Could you check a few things on this model? Use its own coordinates, in mm. Face numbers are marked on the shaded views. A direction names the side the tool comes from. Give positions to 0.01 mm unless a question says otherwise; leave off trailing zeros. Loops run counter-clockwise (first coordinate to the right, second up) from the corner with the lowest first, then second, coordinate; pieces in that order, holes last. Notation, with made-up numbers: M 0.5,-9.5 L 8.5,-9.5 A19 cw 8.5,-2.5 Z; hole C -8.75,1.5 d9. An arc over 180 degrees is marked long. Write each question's results on one line, items separated by ' | '. Start each with the question number.
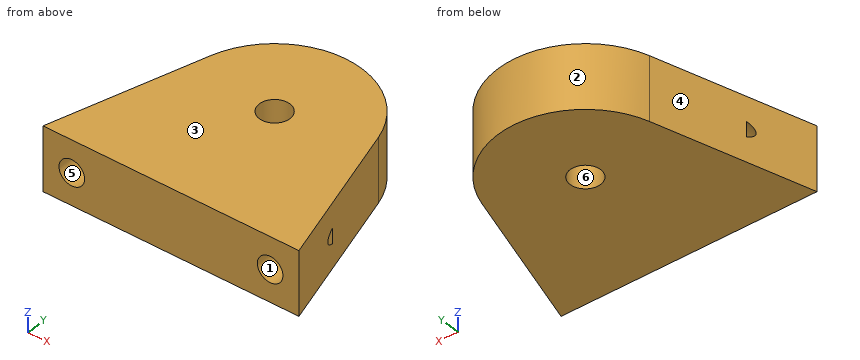
from build123d import *

# Parameters (mm, degrees)
SKETCH2_R           = 2.3876
BOSS_EXTRUDE1_DEPTH = 5
SKETCH3_R           = 2
CUT_EXTRUDE1_DEPTH  = 10


with BuildPart() as part:
    # Sketch2 → Boss-Extrude1 (new body, symmetric)
    with BuildSketch(Plane.XY):
        with BuildLine():
            Line((-20, 0), (20, 0))
            Line((20, 0), (13.124848139, 23.792582213))
            ThreePointArc((13.124848139, 23.792582213), (0, 33.661819737), (-13.124848139, 23.792582213))
            Line((-13.124848139, 23.792582213), (-20, 0))
        make_face()
        with Locations((0, 20)):
            Circle(SKETCH2_R, mode=Mode.SUBTRACT)
    extrude(amount=BOSS_EXTRUDE1_DEPTH, both=True)

    # Sketch3 → Cut-Extrude1 (cut)
    with BuildSketch(Plane(origin=(0, 0, 0), x_dir=(-1, 0, 0), z_dir=(0, -1, 0))):
        with Locations((15.5, 0)):
            Circle(SKETCH3_R)
        with Locations((-15.5, 0)):
            Circle(SKETCH3_R)
    extrude(amount=-CUT_EXTRUDE1_DEPTH, mode=Mode.SUBTRACT)


solid = part.part
1) If we section it at B-B on z = 3: Write out the boundary of the cut face in (x, y).
2) If we section it at A-A on z = 0: Write out the boundary of the cut face in (x, y), plus the area to 3 significant figures.
3) If we section it at C-C on y = 20: Write out the boundary of the cut face in (x, z).
4) Which directions (+Z, -Z, +X, -X, +Y, -Y) give clear straight access to the entire face, cutting with the end or side of a thin tool? Please do the marked faces 1 and 2.
5) Thinking about a two-plate mould opening in X: for the marked faces 3, 4, 5 and 6, which applies, pulls with the +X half, pulls with the -X half, needs draft (parallel to the pull), parting line crosses it, or undercut?
6) If we section it at D-D on y = 8: Write out the boundary of the cut face in (x, z), plus the area to 3 significant figures.
7) Please list where these lines run through material, in increasing order: line 1 (X direction, y = 2, z = -1.5); line 2 (Z direction, x = -15.5, y = 3); line 3 (X direction, y = 5.5, z = 0). Write a range as from..to.
8) I'm going to push flat-ended pins straight in: P1, Ø5, axis at y = 21, z = -3.5, coming from the +X side; P2, Ø2, axis at y = 17.5, z = 0, coming from the +X side; P3, Ø5, axis at x = 12.5, z = 3, coming from the +Y side. Where does each tip first touch, or does it pass through?
Calculated:
1) outline: M -20,0 L 20,0 L 13.12,23.79 A13.66 ccw -13.12,23.79 Z; hole C 0,20 d4.78
2) outline: M -20,0 L -17.5,0 L -17.5,8.65 Z; M -17.11,10 L -13.5,10 L -13.5,0 L 13.5,0 L 13.5,10 L 17.11,10 L 13.12,23.79 A13.66 ccw -13.12,23.79 Z; M 17.5,0 L 20,0 L 17.5,8.65 Z; hole C 0,20 d4.78 | area: 882 mm2
3) outline: M -14.22,-5 L -2.39,-5 L -2.39,5 L -14.22,5 Z; M 2.39,-5 L 14.22,-5 L 14.22,5 L 2.39,5 Z
4) face 1: -Y | face 2: +Z, -Z, +Y
5) face 3: needs draft | face 4: pulls with the -X half | face 5: undercut | face 6: undercut
6) outline: M -17.69,-5 L 17.69,-5 L 17.69,5 L -17.69,5 Z; hole C -15.5,0 d4; hole C 15.5,0 d4 | area: 329 mm2
7) line 1: x = -19.42..-16.82, -14.18..14.18, 16.82..19.42 | line 2: z = -5..-2, 2..5 | line 3: x = -18.41..-17.5, -13.5..13.5, 17.5..18.41
8) P1: stops at x = 14.65 | P2: stops at x = 15.23 | P3: stops at y = 29.31
